Input: part model. Units: mm. Frame: model coordinates. A direction names the side the tool comes from. Coordinates: 2 decimals unless noted, no trailing zeros. Loops run counter-clockwise (first coordinate to the right, second up) from the corner with the lowest first, then second, coordinate; pieces in that order, holes last.
Item 1: Section B-B on z = 0. Return loops of the section in (x, y), and give its area (3 significant figures).
Item 2: Ray query, line 1 along X through (y, z) = (7.75, 0); line 2 along X through (y, z) = (5.75, 1); line 3 along X through (y, z) = (8, -25). Return the intervals inside material, ascending.
Item 3: Section A-A on x = -16.5. Return loops of the section in (y, z).
Item 4: Pull-direction query (Z, two-part tool) for faces 3 (the flat face through (-1, 10, 0)), 4 (the cylindrical face through (60, 5, 27)), 5 (the cylindrical face through (9.106, 8.422, 17.008)); classes: released by +Z, released by -Z, zero draft, split by the parting line, or undercut.
Item 5: Reachability of faces 1 (the flat face through (7, 6.8, -13)), 2 (the flat face through (-1, 0, 0)) from +Z, -Z, +X, -X, +Y, -Y: full face, straight path, thin tool, end or side. Return the list, or none.
Item 6: Contact query for a flat-ended pin moving along its axis: P1, Ø3, axis at x = -15.5, z = 0, coming from the +Y side. Output: stop coordinate, or through.
Item 7: Section C-C on x = 8.25. Return loops of the section in (y, z), and give its area (3 significant figures).
```python
from build123d import *

# Parameters (mm, degrees)
SKIZZE1_W                       = 124
SKIZZE1_H                       = 56
AUFSATZ_LINEAR_AUSTRAGEN1_DEPTH = 10
VERRUNDUNG1_R                   = 5
SCHNITT_LINEAR_AUSTRAGEN1_REACH = 70.76
SKIZZE2_R                       = 1.55
SKIZZE3_R                       = 2.85
SCHNITT_LINEAR_AUSTRAGEN2_DEPTH = 3.2


with BuildPart() as part:
    # Skizze1 → Aufsatz-Linear austragen1 (new body)
    with BuildSketch(Plane(origin=(0, 0, 0), x_dir=(1, 0, 0), z_dir=(0, 1, 0))):
        Rectangle(SKIZZE1_W, SKIZZE1_H)
    extrude(amount=AUFSATZ_LINEAR_AUSTRAGEN1_DEPTH)

    # Verrundung1
    verrundung1_edges = [part.edges().sort_by_distance(p)[0] for p in [
        (62, 5, -28),
        (62, 5, 28),
        (-62, 5, 28),
        (-62, 5, -28),
    ]]
    fillet(verrundung1_edges, radius=VERRUNDUNG1_R)

    # Skizze2 → Schnitt-Linear austragen1 (cut, up to next)
    with BuildSketch(Plane(origin=(0, 10, 0), x_dir=(1, 0, 0), z_dir=(0, 1, 0)), mode=Mode.PRIVATE) as schnitt_linear_austragen1_sk1:
        with Locations(Location((-16.5, 0, 0), (0, 0, 270))):
            Circle(SKIZZE2_R)
    schnitt_linear_austragen1_tool1 = extrude(schnitt_linear_austragen1_sk1.sketch, amount=-SCHNITT_LINEAR_AUSTRAGEN1_REACH, mode=Mode.PRIVATE) & part.part
    # Skizze2 → Schnitt-Linear austragen1 (cut, up to next)
    with BuildSketch(Plane(origin=(0, 10, 0), x_dir=(1, 0, 0), z_dir=(0, 1, 0)), mode=Mode.PRIVATE) as schnitt_linear_austragen1_sk2:
        with Locations(Location((8.25, 14.289419162, 0), (0, 0, 270))):
            Circle(SKIZZE2_R)
    schnitt_linear_austragen1_tool2 = extrude(schnitt_linear_austragen1_sk2.sketch, amount=-SCHNITT_LINEAR_AUSTRAGEN1_REACH, mode=Mode.PRIVATE) & part.part
    # Skizze2 → Schnitt-Linear austragen1 (cut, up to next)
    with BuildSketch(Plane(origin=(0, 10, 0), x_dir=(1, 0, 0), z_dir=(0, 1, 0)), mode=Mode.PRIVATE) as schnitt_linear_austragen1_sk3:
        with Locations(Location((8.25, -14.289419162, 0), (0, 0, 270))):
            Circle(SKIZZE2_R)
    schnitt_linear_austragen1_tool3 = extrude(schnitt_linear_austragen1_sk3.sketch, amount=-SCHNITT_LINEAR_AUSTRAGEN1_REACH, mode=Mode.PRIVATE) & part.part
    add(schnitt_linear_austragen1_tool1.solids().sort_by_distance((-16.5, 10, 0))[0], mode=Mode.SUBTRACT)
    add(schnitt_linear_austragen1_tool2.solids().sort_by_distance((8.25, 10, -14.289419))[0], mode=Mode.SUBTRACT)
    add(schnitt_linear_austragen1_tool3.solids().sort_by_distance((8.25, 10, 14.289419))[0], mode=Mode.SUBTRACT)

    # Skizze3 → Schnitt-Linear austragen2 (cut)
    with BuildSketch(Plane(origin=(0, 10, 0), x_dir=(1, 0, 0), z_dir=(0, 1, 0))):
        with Locations(Location((8.25, 14.289419162, 0), (0, 0, 270))):
            Circle(SKIZZE3_R)
        with Locations(Location((-16.5, 0, 0), (0, 0, 270))):
            Circle(SKIZZE3_R)
        with Locations(Location((8.25, -14.289419162, 0), (0, 0, 270))):
            Circle(SKIZZE3_R)
    extrude(amount=-SCHNITT_LINEAR_AUSTRAGEN2_DEPTH, mode=Mode.SUBTRACT)


solid = part.part
```
Results found:
1. outline: (-62, 0) - (-18.05, 0) - (-18.05, 6.8) - (-19.35, 6.8) - (-19.35, 10) - (-62, 10) - close; (-14.95, 0) - (62, 0) - (62, 10) - (-13.65, 10) - (-13.65, 6.8) - (-14.95, 6.8) - close
1. area: 1,200 mm2
2. line 1: x = -62 to -19.35, -13.65 to 62
2. line 2: x = -62 to -17.68, -15.32 to 62
2. line 3: x = -61.58 to 61.58
3. outline: (0, -28) - (10, -28) - (10, -2.85) - (6.8, -2.85) - (6.8, -1.55) - (0, -1.55) - close; (0, 1.55) - (6.8, 1.55) - (6.8, 2.85) - (10, 2.85) - (10, 28) - (0, 28) - close
4. face 3: zero draft
4. face 4: released by +Z
4. face 5: undercut
5. face 1: +Y
5. face 2: +Z, -Z, +X, -X, -Y
6. P1: stops at y = 6.8
7. outline: (0, -28) - (10, -28) - (10, -17.14) - (6.8, -17.14) - (6.8, -15.84) - (0, -15.84) - close; (0, -12.74) - (6.8, -12.74) - (6.8, -11.44) - (10, -11.44) - (10, 11.44) - (6.8, 11.44) - (6.8, 12.74) - (0, 12.74) - close; (0, 15.84) - (6.8, 15.84) - (6.8, 17.14) - (10, 17.14) - (10, 28) - (0, 28) - close
7. area: 481 mm2
